Source: CAD feature listing. Evaluate the final solid. Frame: model axes, mm. Face numbers are marked on the shaded views. Round coordinates to 2 decimals unless told otherwise and drop trailing zeros. Write each loop counter-clockwise with the first axis right and the second up, starting at its lowest first coordinate (ties: lowest second). Pieces come first, ordered by that corner, then holes. Notation, with made-up numbers: (40.5, 27) - (90.5, 27) arc R22 ccw to (90.5, 62) - close; hole circle Ø4 at (-25.5, 64.5). An arc over 180 degrees is marked (long way). Write item = value, one per line. Start each with the question number.
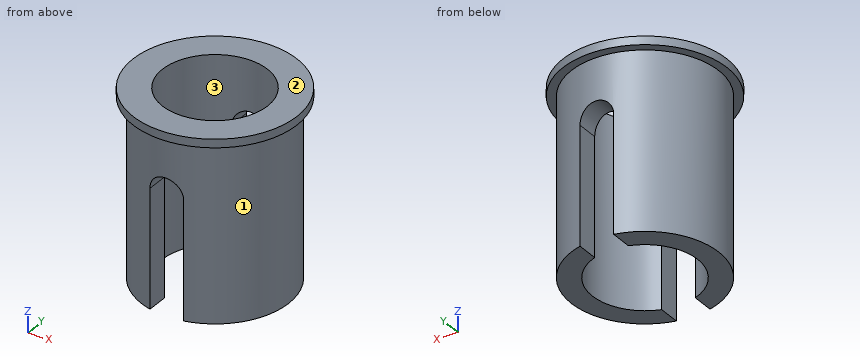
```python
from build123d import *

# Parameters (mm, degrees)
SKETCH_1_R               = 17.5
SKETCH_1_R_2             = 12.5
EXTRUDE_1_DEPTH          = 2
EXTRUDE_1_DEPTH_BACK     = 42
SKETCH_2_R               = 19.5
SKETCH_2_R_2             = 17.5
EXTRUDE_2_DEPTH          = 2
CUT_EXTRUDE_1_DEPTH      = 20.5
CUT_EXTRUDE_1_DEPTH_BACK = 20.5


with BuildPart() as part:
    # Эскиз1 → Бобышка-Вытянуть1 (new body, two sides)
    with BuildSketch(Plane.XY) as extrude_1_sk:
        Circle(SKETCH_1_R)
        Circle(SKETCH_1_R_2, mode=Mode.SUBTRACT)
    extrude(amount=EXTRUDE_1_DEPTH)
    extrude(extrude_1_sk.sketch, amount=-EXTRUDE_1_DEPTH_BACK)

    # Эскиз2 → Бобышка-Вытянуть2 (add)
    with BuildSketch(Plane.XY.offset(2)):
        Circle(SKETCH_2_R)
        Circle(SKETCH_2_R_2, mode=Mode.SUBTRACT)
    extrude(amount=-EXTRUDE_2_DEPTH)

    # Эскиз3 → Вырез-Вытянуть1 (cut, two sides)
    with BuildSketch(Plane(origin=(0, 0, 0), x_dir=(1, 0, 0), z_dir=(0, 1, 0))) as cut_extrude_1_sk:
        with BuildLine():
            Line((4, 42), (4, 14))
            ThreePointArc((4, 14), (0, 10), (-4, 14))
            Line((-4, 14), (-4, 42))
            ThreePointArc((-4, 42), (0, 46), (4, 42))
        make_face()
    extrude(amount=CUT_EXTRUDE_1_DEPTH, mode=Mode.SUBTRACT)
    extrude(cut_extrude_1_sk.sketch, amount=-CUT_EXTRUDE_1_DEPTH_BACK, mode=Mode.SUBTRACT)


solid = part.part
```
(1) Section D-D (z = -11). Return the cut outline in (x, y).
(2) Contact query for flat-ended pins moving along their axis: P1, Ø10, axis at y = -12.5, z = -13, coming from the +X side; P2, Ø12, axis at x = -2, z = -15, coming from the -Y side; P3, Ø4, axis at y = 14.5, z = -22, coming from the -X side; P4, Ø3, axis at x = -5, y = -11, coming from the -Z side. Output: stop coordinate, or through.
(3) Section A-A (z = -19.5). Return the cut outline in (x, y), plus the area to 3 significant figures.
(4) Ray query, L1, parallel to X at y = 0, z = -29.5; L2, parallel to X at y = 4.5, z = -1; L3, parallel to Z at x = -4, y = -18. Return the intervals inside material, ascending. Write a range as from..to.
(5) Pull-direction query (X, two-part tool) for the marked faces 1, 2 and 3; classes: +X half, -X half, draft (parallel to the pull), parting line (faces both ways), or undercut.
(6) Section B-B (y = 0). Return the cut outline in (x, z).
(7) Section C-C (x = 2). Return the cut outline in (y, z), plus the area to 3 significant figures.
Solution:
q1.outline = (-2.65, -17.3) - (-2.65, -12.22) arc R12.5 cw to (-2.65, 12.22) - (-2.65, 17.3) arc R17.5 ccw to start; (2.65, -17.3) arc R17.5 ccw to (2.65, 17.3) - (2.65, 12.22) arc R12.5 cw to (2.65, -12.22) - close
q2.P1 = 15.81
q2.P2 = -17.5
q2.P3 = -12.25
q2.P4 = -42
q3.outline = (-4, -17.04) - (-4, -11.84) arc R12.5 cw to (-4, 11.84) - (-4, 17.04) arc R17.5 ccw to start; (4, -17.04) arc R17.5 ccw to (4, 17.04) - (4, 11.84) arc R12.5 cw to (4, -11.84) - close
q3.area = 390 mm^2
q4.L1 = -17.5..-12.5, 12.5..17.5
q4.L2 = -16.91..-11.66, 11.66..16.91
q4.L3 = 0..2
q5.face_1 = parting line
q5.face_2 = draft
q5.face_3 = undercut
q6.outline = (-19.5, 0) - (-17.5, 0) - (-17.5, -42) - (-12.5, -42) - (-12.5, 2) - (-19.5, 2) - close; (12.5, -42) - (17.5, -42) - (17.5, 0) - (19.5, 0) - (19.5, 2) - (12.5, 2) - close
q7.outline = (-19.4, 0) - (-17.39, 0) - (-17.39, -10.54) - (-12.34, -10.54) - (-12.34, 2) - (-19.4, 2) - close; (12.34, -10.54) - (17.39, -10.54) - (17.39, 0) - (19.4, 0) - (19.4, 2) - (12.34, 2) - close
q7.area = 135 mm^2
